For this review, take the finished solid that the model builds, in its own axes (mm). A direction names the side the tool comes from. Coordinates: 2 decimals unless noted, no trailing zeros. Write each loop counter-clockwise with the first axis right and the second up, starting at its lowest first coordinate (ties: lowest second). Pieces come first, ordered by that corner, then holes. Notation, with made-up numbers: M -39.5,30 L 17.5,30 A17 cw 17.5,57 Z; hole C 15,23.5 d11. An arc over 180 degrees is marked long. Return JSON: item names as keys, results as strings.
```python
from build123d import *

# Parameters (mm, degrees)
SKETCH1_W                               = 94
SKETCH1_H                               = 63.5
BOSS_EXTRUDE1_DEPTH                     = 76.2
SKETCH2_W                               = 82.000024
SKETCH2_H                               = 51.500024
CUT_EXTRUDE1_DEPTH                      = 70.2
SKETCH7_R                               = 31.95
CUT_EXTRUDE4_DEPTH                      = 4
SKETCH8_R                               = 12.55
CUT_EXTRUDE5_DEPTH                      = 2
SKETCH14_W                              = 8
SKETCH14_H                              = 9.3
BOSS_EXTRUDE2_DEPTH                     = 42.2
BOSS_EXTRUDE3_DEPTH                     = 22
F_1_0MM_DOWEL_HOLE1_D                   = 3.4
F_1_0MM_DOWEL_HOLE1_DEPTH               = 10.5
F_1_0MM_DOWEL_HOLE1_TIP                 = 1.021463052
F_1_0MM_DOWEL_HOLE2_D                   = 4
F_1_0MM_DOWEL_HOLE2_DEPTH               = 5.3
F_1_0MM_DOWEL_HOLE2_TIP                 = 1.201721238
FILLET1_R                               = 5
BOSS_EXTRUDE4_DEPTH                     = 70.2
CBORE_FOR_M5_HEX_HEAD_BOLT1_D           = 6.5
CBORE_FOR_M5_HEX_HEAD_BOLT1_DEPTH       = 10.75
CBORE_FOR_M5_HEX_HEAD_BOLT1_CBORE_D     = 9.05
CBORE_FOR_M5_HEX_HEAD_BOLT1_CBORE_DEPTH = 1
CBORE_FOR_M5_HEX_HEAD_BOLT1_TIP         = 1.952797012
SKETCH49_R                              = 15.875
CUT_EXTRUDE7_DEPTH                      = 5.999988
BOSS_EXTRUDE5_START                     = 10
SKETCH51_R                              = 18.875
SKETCH51_R_2                            = 15.875
BOSS_EXTRUDE5_DEPTH                     = 10
SKETCH52_R                              = 2.75
CUT_EXTRUDE8_DEPTH                      = 124.940865436
CUT_EXTRUDE9_DEPTH                      = 1.999988
FILLET2_R                               = 3
FILLET3_R                               = 2


with BuildPart() as part:
    # Sketch1 → Boss-Extrude1 (new body)
    with BuildSketch(Plane(origin=(0, 0, 0), x_dir=(1, 0, 0), z_dir=(0, 1, 0))):
        with Locations((47, 0)):
            Rectangle(SKETCH1_W, SKETCH1_H)
    extrude(amount=BOSS_EXTRUDE1_DEPTH)

    # Sketch2 → Cut-Extrude1 (cut)
    with BuildSketch(Plane(origin=(0, 76.2, 0), x_dir=(1, 0, 0), z_dir=(0, 1, 0))):
        with Locations((47, 0)):
            Rectangle(SKETCH2_W, SKETCH2_H)
    extrude(amount=-CUT_EXTRUDE1_DEPTH, mode=Mode.SUBTRACT)

    # Sketch7 → Cut-Extrude4 (cut)
    with BuildSketch(Plane(origin=(0, 0, -31.75), x_dir=(-1, 0, 0), z_dir=(0, 0, -1))):
        with Locations((-38.1, 38.1)):
            Circle(SKETCH7_R)
    extrude(amount=-CUT_EXTRUDE4_DEPTH, mode=Mode.SUBTRACT)

    # Sketch8 → Cut-Extrude5 (cut)
    with BuildSketch(Plane.XY.offset(-25.750012)):
        with Locations((38.1, 38.1)):
            Circle(SKETCH8_R)
    extrude(amount=-CUT_EXTRUDE5_DEPTH, mode=Mode.SUBTRACT)

    # Sketch14 → Boss-Extrude2 (add)
    with BuildSketch(Plane(origin=(0, 6, 0), x_dir=(1, 0, 0), z_dir=(0, 1, 0))):
        with Locations((23.999988, 4.450012)):
            Rectangle(SKETCH14_W, SKETCH14_H)
        with Locations((72.499988, 4.450012)):
            Rectangle(SKETCH14_W, SKETCH14_H)
    extrude(amount=BOSS_EXTRUDE2_DEPTH)

    # Sketch15 → Boss-Extrude3 (add)
    with BuildSketch(Plane(origin=(0, 28, 0), x_dir=(1, 0, 0), z_dir=(0, 1, 0))):
        Polygon((27.999988, 9.100012), (68.499988, 9.100012), (68.499988, -0.199988), (76.499988, -0.199988), (76.499988, -11.199988), (19.999988, -11.199988), (19.999988, -0.199988), (27.999988, -0.199988), align=None)
    extrude(amount=-BOSS_EXTRUDE3_DEPTH)

    # Ø1.0mm Dowel Hole1
    with Locations(Plane(origin=(0, 28, 0), x_dir=(1, 0, 0), z_dir=(0, 1, 0))):
        with Locations((22.999988, -5.699988), (73.499988, -5.699988)):
            Hole(F_1_0MM_DOWEL_HOLE1_D / 2, depth=F_1_0MM_DOWEL_HOLE1_DEPTH)
            with Locations((0, 0, -(F_1_0MM_DOWEL_HOLE1_DEPTH + F_1_0MM_DOWEL_HOLE1_TIP / 2))):  # 118° drill point
                Cone(0, F_1_0MM_DOWEL_HOLE1_D / 2, F_1_0MM_DOWEL_HOLE1_TIP, mode=Mode.SUBTRACT)

    # Ø1.0mm Dowel Hole2
    with Locations(Plane(origin=(0, 0, -9.100012), x_dir=(-1, 0, 0), z_dir=(0, 0, -1))):
        with Locations((-72.499988, 42.43), (-72.499988, 33.72), (-23.999988, 42.43), (-23.999988, 33.72)):
            Hole(F_1_0MM_DOWEL_HOLE2_D / 2, depth=F_1_0MM_DOWEL_HOLE2_DEPTH)
            with Locations((0, 0, -(F_1_0MM_DOWEL_HOLE2_DEPTH + F_1_0MM_DOWEL_HOLE2_TIP / 2))):  # 118° drill point
                Cone(0, F_1_0MM_DOWEL_HOLE2_D / 2, F_1_0MM_DOWEL_HOLE2_TIP, mode=Mode.SUBTRACT)

    # Fillet1
    fillet1_edges = [part.edges().sort_by_distance(p)[0] for p in [
        (47, 0, -31.75),
        (94, 0, 0),
        (47, 0, 31.75),
        (0, 0, 0),
        (0, 38.1, -31.75),
        (94, 38.1, -31.75),
        (94, 38.1, 31.75),
        (0, 38.1, 31.75),
    ]]
    fillet(fillet1_edges, radius=FILLET1_R)

    # Sketch44 → Boss-Extrude4 (add)
    with BuildSketch(Plane(origin=(0, 76.2, 0), x_dir=(1, 0, 0), z_dir=(0, 1, 0))):
        with BuildLine():
            Line((8.499988, 17.250012), (5.999988, 17.250012))
            Line((5.999988, 17.250012), (5.999988, 25.750012))
            Line((5.999988, 25.750012), (14.499988, 25.750012))
            Line((14.499988, 25.750012), (14.499988, 23.250012))
            ThreePointArc((14.499988, 23.250012), (12.742628687, 19.007371313), (8.499988, 17.250012))
        make_face()
        with BuildLine():
            Line((8.499988, -17.250012), (5.999988, -17.250012))
            Line((5.999988, -17.250012), (5.999988, -25.750012))
            Line((5.999988, -25.750012), (14.499988, -25.750012))
            Line((14.499988, -25.750012), (14.499988, -23.250012))
            ThreePointArc((14.499988, -23.250012), (12.742628687, -19.007371313), (8.499988, -17.250012))
        make_face()
        with BuildLine():
            Line((79.500012, -23.250012), (79.500012, -25.750012))
            Line((79.500012, -25.750012), (88.000012, -25.750012))
            Line((88.000012, -25.750012), (88.000012, -17.250012))
            Line((88.000012, -17.250012), (85.500012, -17.250012))
            ThreePointArc((85.500012, -17.250012), (81.257371313, -19.007371313), (79.500012, -23.250012))
        make_face()
        with BuildLine():
            Line((79.500012, 23.250012), (79.500012, 25.750012))
            Line((79.500012, 25.750012), (88.000012, 25.750012))
            Line((88.000012, 25.750012), (88.000012, 17.250012))
            Line((88.000012, 17.250012), (85.500012, 17.250012))
            ThreePointArc((85.500012, 17.250012), (81.257371313, 19.007371313), (79.500012, 23.250012))
        make_face()
    extrude(amount=-BOSS_EXTRUDE4_DEPTH)

    # CBORE for M5 Hex Head Bolt1
    with Locations(Plane(origin=(0, 76.2, 0), x_dir=(1, 0, 0), z_dir=(0, 1, 0))):
        with Locations((8.499988, 23.250012), (8.499988, -23.250012), (85.500012, -23.250012), (85.500012, 23.250012)):
            CounterBoreHole(CBORE_FOR_M5_HEX_HEAD_BOLT1_D / 2, CBORE_FOR_M5_HEX_HEAD_BOLT1_CBORE_D / 2, CBORE_FOR_M5_HEX_HEAD_BOLT1_CBORE_DEPTH, depth=CBORE_FOR_M5_HEX_HEAD_BOLT1_DEPTH)
            with Locations((0, 0, -(CBORE_FOR_M5_HEX_HEAD_BOLT1_DEPTH + CBORE_FOR_M5_HEX_HEAD_BOLT1_TIP / 2))):  # 118° drill point
                Cone(0, CBORE_FOR_M5_HEX_HEAD_BOLT1_D / 2, CBORE_FOR_M5_HEX_HEAD_BOLT1_TIP, mode=Mode.SUBTRACT)

    # Sketch49 → Cut-Extrude7 (cut)
    with BuildSketch(Plane(origin=(94, 0, 0), x_dir=(0, 0, -1), z_dir=(1, 0, 0))):
        with Locations((0, 40.6)):
            Circle(SKETCH49_R)
    extrude(amount=-CUT_EXTRUDE7_DEPTH, mode=Mode.SUBTRACT)

    # Sketch51 → Boss-Extrude5 (add)
    with BuildSketch(Plane(origin=(94, 0, 0), x_dir=(0, 0, -1), z_dir=(1, 0, 0)).offset(BOSS_EXTRUDE5_START)):
        with Locations(Location((0, 40.6, 0), (0, 0, 180))):
            Circle(SKETCH51_R)
        with Locations((0, 40.6)):
            Circle(SKETCH51_R_2, mode=Mode.SUBTRACT)
    extrude(amount=-BOSS_EXTRUDE5_DEPTH)

    # Sketch52 → Cut-Extrude8 (cut, through all)
    with BuildSketch(Plane(origin=(0, 59.475, 0), x_dir=(-1, 0, 0), z_dir=(0, 1, 0))):
        with Locations(Location((-99, 0, 0), (0, 0, 90))):
            Circle(SKETCH52_R)
    extrude(amount=-CUT_EXTRUDE8_DEPTH, mode=Mode.SUBTRACT)

    # Sketch53 → Cut-Extrude9 (cut)
    with BuildSketch(Plane(origin=(0, 0, -27.75), x_dir=(-1, 0, 0), z_dir=(0, 0, -1))):
        with BuildLine():
            Line((-38.1, 61.27), (-38.1, 14.93))
            ThreePointArc((-38.1, 14.93), (-14.93, 38.1), (-38.1, 61.27))
        make_face()
    extrude(amount=-CUT_EXTRUDE9_DEPTH, mode=Mode.SUBTRACT)

    # Fillet2
    fillet2_edges = [part.edges().sort_by_distance(p)[0] for p in [
        (38.1, 14.93, -26.750006),
        (38.1, 61.27, -26.750006),
    ]]
    fillet(fillet2_edges, radius=FILLET2_R)

    # Fillet3
    # the kernel refuses this fillet: 2 mm, written as the material it takes off along each edge
    with BuildSketch(Plane(origin=(38.1, 58.045648648, -25.750012), x_dir=(0, 0, -1), z_dir=(0, -1, 0)), Plane(origin=(38.1, 30.55, -25.750012), x_dir=(0, 0, -1), z_dir=(0, -1, 0))) as fillet3_piece_1:
        with BuildLine():
            CenterArc((2, 2), FILLET3_R, 180, 89.999656225)
            Line((0, 2), (-0.04, 2))
            Line((-0.04, 2), (-0.04, 0))
            Line((-0.04, 0), (0, -0.04))
            Line((0, -0.04), (1.99998776, -0.04))
            Line((1.99998776, -0.04), (1.999988, 0))
        make_face()
    extrude(amount=12.395648648, mode=Mode.SUBTRACT)
    with BuildSketch(Plane(origin=(35.1, 58.045648648, -25.750012), x_dir=(-0.14873574615765991, 0.988876978099361, 0), z_dir=(-0.988876978099361, -0.14873574615765991, 0))) as fillet3_piece_2:
        with BuildLine():
            CenterArc((5, 2), FILLET3_R, 180.000343775, 89.999656225)
            Line((5, 0), (5, -0.04))
            Line((5, -0.04), (3, -0.04))
            Line((3, -0.04), (2.96, 0))
            Line((2.96, 0), (2.96, 1.99998776))
            Line((2.96, 1.99998776), (3, 1.999988))
        make_face()
    revolve(axis=Axis((35.1, 58.045648648, -25.750012), (0, 0, -1)), revolution_arc=98.553668311, mode=Mode.SUBTRACT)
    with BuildSketch(Plane(origin=(35.1, 18.154351352, -25.750012), x_dir=(1, 0, 0), z_dir=(0, 1, 0))) as fillet3_piece_3:
        with BuildLine():
            CenterArc((5, 2), FILLET3_R, 180.000343775, 89.999656225)
            Line((5, 0), (5, -0.04))
            Line((5, -0.04), (3, -0.04))
            Line((3, -0.04), (2.96, 0))
            Line((2.96, 0), (2.96, 1.99998776))
            Line((2.96, 1.99998776), (3, 1.999988))
        make_face()
    revolve(axis=Axis((35.1, 18.154351352, -25.750012), (0, 0, -1)), revolution_arc=98.553668311, mode=Mode.SUBTRACT)
    with BuildSketch(Plane(origin=(38.1, 38.1, -25.750012), x_dir=(-0.14873574615765983, -0.988876978099361, 0), z_dir=(0.988876978099361, -0.14873574615765983, 0))) as fillet3_piece_4_section:
        with BuildLine():
            CenterArc((25.17, 2), FILLET3_R, 180.000343775, 89.999656225)
            Line((25.17, 0), (25.17, -0.04))
            Line((25.17, -0.04), (23.17, -0.04))
            Line((23.17, -0.04), (23.13, 0))
            Line((23.13, 0), (23.13, 1.99998776))
            Line((23.13, 1.99998776), (23.17, 1.999988))
        make_face()
    fillet3_piece_4 = revolve(axis=Axis((38.1, 38.1, -25.750012), (0, 0, -1)), revolution_arc=162.892663379, mode=Mode.PRIVATE)
    fillet3_piece_4 = split(fillet3_piece_4, bisect_by=Plane(origin=(14.499988, 19.260781235, -27.221962955), z_dir=(1, 0, 0)), keep=Keep.TOP, mode=Mode.PRIVATE)
    add(fillet3_piece_4, mode=Mode.SUBTRACT)


solid = part.part
```
1. We need section B-B (x = 56). State the section outline as (y, z) points.
Checks:
{"outline": "M 0,-26.75 A5 ccw 5,-31.75 L 11.64,-31.75 L 11.64,-27.75 L 64.56,-27.75 L 64.56,-31.75 L 76.2,-31.75 L 76.2,-25.75 L 6,-25.75 L 6,-9.1 L 28,-9.1 L 28,11.2 L 6,11.2 L 6,25.75 L 76.2,25.75 L 76.2,31.75 L 5,31.75 A5 ccw 0,26.75 Z"}
2. Wall thickness on L1, parallel to Z at x = 56.5, y = 15.5; L2, parallel to X at y = 10, z = -1; L3, parallel to X at y = 42.43, z = -7.1: over which ranges is each line inside the solid? List them lowest first. Write a range as from..to.
Checks:
{"L1": "-27.75..-25.75, -9.1..11.2, 25.75..31.75", "L2": "0..6, 20..76.5, 88..94", "L3": "0..6, 20..22, 26..28, 68.5..70.5, 74.5..76.5"}
3. Draft analysis for pull direction X (two halves, no side actions). For faces 1 (the face through (46, 40, 31.75)), 2 (the face through (4.909, 75.707, -20.497)), 3 (the face through (104, 25, -4)), state which applies: +X half, -X half, draft (parallel to the pull), parting line (faces both ways), or undercut.
Checks:
{"face 1": "draft", "face 2": "undercut", "face 3": "+X half"}
4. We need section A-A (z = -12.5). State the section outline as (x, y) points.
Checks:
{"outline": "M 0,5 A5 ccw 5,0 L 89,0 A5 ccw 94,5 L 94,26.46 L 104,26.46 L 104,30.81 L 88,30.81 L 88,6 L 6,6 L 6,76.2 L 0,76.2 Z; M 88,50.39 L 104,50.39 L 104,54.74 L 94,54.74 L 94,76.2 L 88,76.2 Z"}
5. Clearance check with flat-ended pins moving along their axes: pin 1 Ø8.5 at (x, z) = (85.5, 23.25) entering from +Y; pin 2 Ø3.5 at (y, z) = (49.5, -25) entering from +X; pin 3 Ø3.5 at (x, y) = (24, 42.43) entering from -Z. State where each tip first meets the part, or that it passes through.
Checks:
{"pin 1": "y = 75.2", "pin 2": "x = 94", "pin 3": "z = -3.65"}
6. We need section C-C (y = 38.1). Give the number of separate pieces and of enclosed holes in the cut face, plus the area to 3 significant figures.
Checks:
{"separate pieces": "4", "enclosed holes": "0", "area": "1,680 mm2"}
7. For faces 4 (the face through (80.98, 75.71, 23.05)), 5 (the face through (99.07, 59.026, -4.092)), 6 (the face through (50.647, 37.824, -26.736)), 7 (the face through (24, 38, 0.2)), list the 3-axis set-ups (+Z, -Z, +X, -X, +Y, -Y) from which the entire face can be reached by the end or side of a thin tool; tool diameter is ignored.
Checks:
{"face 4": "+Y", "face 5": "+X", "face 6": "-Z", "face 7": "+X, +Y"}
